```python
from build123d import *

# Parameters (mm, degrees)
SKETCH1_W           = 25.4
SKETCH1_H           = 152.4
SKETCH1_R           = 3.175
BOSS_EXTRUDE1_DEPTH = 25.4
SKETCH3_R           = 6.35
CUT_EXTRUDE5_DEPTH  = 26.4
SKETCH5_W           = 21.59
SKETCH5_H           = 21.59
SKETCH5_H_2         = 25.4
CUT_EXTRUDE6_DEPTH  = 19.05


with BuildPart() as part:
    # Sketch1 → Boss-Extrude1 (new body)
    with BuildSketch(Plane.XY):
        with Locations((12.7, 76.2)):
            Rectangle(SKETCH1_W, SKETCH1_H)
        with Locations((12.7, 63.5)):
            Circle(SKETCH1_R, mode=Mode.SUBTRACT)
    extrude(amount=BOSS_EXTRUDE1_DEPTH)

    # Sketch3 → Cut-Extrude5 (cut, through all)
    with BuildSketch(Plane(origin=(25.4, 0, 0), x_dir=(0, 0, -1), z_dir=(1, 0, 0))):
        with Locations((-12.7, 120.65254)):
            Circle(SKETCH3_R)
        with Locations((-12.7, 6.35254)):
            Circle(SKETCH3_R)
    extrude(amount=-CUT_EXTRUDE5_DEPTH, mode=Mode.SUBTRACT)

    # Sketch5 → Cut-Extrude6 (cut)
    with BuildSketch(Plane(origin=(25.4, 0, 0), x_dir=(0, 0, -1), z_dir=(1, 0, 0))):
        with Locations((-12.7, 6.35254)):
            Rectangle(SKETCH5_W, SKETCH5_H)
        with Locations((-12.7, 120.65254)):
            Rectangle(SKETCH5_W, SKETCH5_H_2)
    extrude(amount=-CUT_EXTRUDE6_DEPTH, mode=Mode.SUBTRACT)


solid = part.part
```
CAD build for the part. Positions are in the model's coordinates, mm. A direction names the side the tool comes from. Round coordinates to 2 decimals unless told otherwise and drop trailing zeros. Write each loop counter-clockwise with the first axis right and the second up, starting at its lowest first coordinate (ties: lowest second). Pieces come first, ordered by that corner, then holes. Notation, with made-up numbers: M 25,-6.5 L 36,-6.5 A21 cw 36,-0.5 Z; hole C -33.5,47 d10. An arc over 180 degrees is marked long. One line per question, with ' | ' between items.
1. Cut at A-A on x = 12.7. Write the cut outline in (y, z) (3 decimals), and give its area (3 significant figures).
Working result:
outline: M 0,0 L 60.325,0 L 60.325,25.4 L 0,25.4 L 0,23.495 L 17.148,23.495 L 17.148,1.905 L 0,1.905 Z; M 66.675,0 L 152.4,0 L 152.4,25.4 L 66.675,25.4 Z; hole M 107.953,1.905 L 133.353,1.905 L 133.353,23.495 L 107.953,23.495 Z | area: 2,790 mm2
2. Cut at B-B on z = 12.7. Count the separate pieces of the cut face and the enclosed holes in it, and give its area (3 significant figures).
Working result:
separate pieces: 3 | enclosed holes: 1 | area: 2,870 mm2
3. Cut at D-D on x = 19. Write the cut outline in (y, z) (3 decimals), and give its area (3 significant figures).
Working result:
outline: M 0,0 L 152.4,0 L 152.4,25.4 L 0,25.4 L 0,23.495 L 17.148,23.495 L 17.148,1.905 L 0,1.905 Z; hole M 107.953,1.905 L 133.353,1.905 L 133.353,23.495 L 107.953,23.495 Z | area: 2,950 mm2
4. Probe L1, parallel to Y at x = 12.7, z = 5.75 (3 decimals); L2, parallel to Z at x = 9, y = 16.5 (3 decimals); L3, parallel to Y at x = 5.25, z = 9.25. List the from-to ranges inside material, lowest first. Write a range as from..to.
Working result:
L1: 17.148..60.325, 66.675..107.953, 133.353..152.4 | L2: 0..1.905, 23.495..25.4 | L3: 0..1.02, 11.68..115.32, 125.98..152.4
5. Cut at C-C on y = 63.5. Write the cut outline in (x, z) (3 decimals), and give its area (3 significant figures).
Working result:
outline: M 0,0 L 9.525,0 L 9.525,25.4 L 0,25.4 Z; M 15.875,0 L 25.4,0 L 25.4,25.4 L 15.875,25.4 Z | area: 484 mm2
6. Mould opens along Y. For faces 4 (the flat face through (16, 17.148, 13)), 5 (the flat face through (16, 8, 1.905)), 6 (the cylindrical face through (10.36, 65.646, 12.522)) say: pulls with the +Y half, pulls with the -Y half, needs draft (parallel to the pull), parting line crosses it, or undercut.
Working result:
face 4: pulls with the -Y half | face 5: needs draft | face 6: undercut
7. Pin check, flat tips, straight feed: pin 1 Ø5 at (y, z) = (11, 9) entering from +X; pin 2 Ø15 at (x, z) = (15.5, 11.5) entering from -Y. Stop position of each tip, or through.
Working result:
pin 1: x = 6.35 | pin 2: y = 17.15
8. Which spindle directions (+Z, -Z, +X, -X, +Y, -Y) get a long thin tool onto all of the face, cutting with end or side? Do faces 1 (the flat face through (13, 77, 0)), 2 (the flat face through (6.35, 13, 15)), 3 (the flat face through (16, 120, 23.495)). Say none if no direction does.
Working result:
face 1: -Z, +X, -X, +Y, -Y | face 2: +X, -Y | face 3: +X
